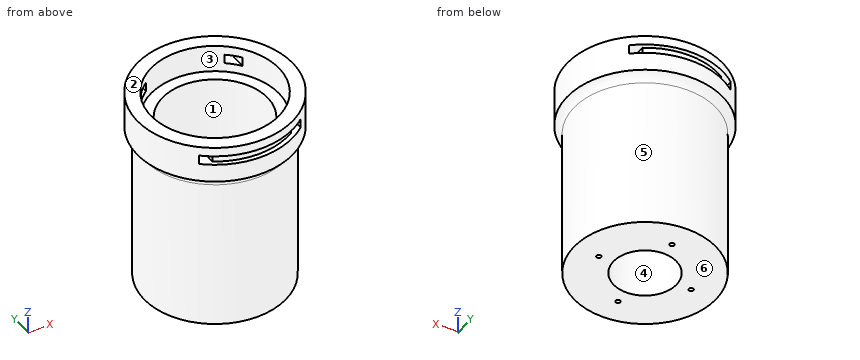
```python
from build123d import *

# Parameters (mm, degrees)
BOSS_EXTRUDE5_DEPTH      = 26
BOSS_EXTRUDE5_DEPTH_BACK = 17
SKETCH1_R                = 15.5
SKETCH3_R                = 5.625
CUT_EXTRUDE2_DEPTH       = 49.264894074
CUT_EXTRUDE3_DEPTH       = 28
CUT_EXTRUDE3_DEPTH_BACK  = 20
SKETCH4_R                = 11.5
CUT_EXTRUDE6_START       = 6
SKETCH7_R                = 11.5
SKETCH7_R_2              = 8.5
CUT_EXTRUDE6_DEPTH       = 18
BOSS_EXTRUDE8_DEPTH      = 6
BOSS_EXTRUDE8_DEPTH_BACK = 2
BOSS_EXTRUDE8_START      = 20
SKETCH12_R               = 17
CUT_EXTRUDE10_START      = 18
SKETCH13_R               = 11.5
CUT_EXTRUDE10_DEPTH      = 18.411862419
FILLET2_R                = 2
CUT_EXTRUDE11_START      = 26
SKETCH14_R               = 14
CUT_EXTRUDE11_DEPTH      = 6
CUT_EXTRUDE14_DEPTH      = 36.411862419
CUT_EXTRUDE14_DEPTH_BACK = 36.411862419
SKETCH15_R               = 0.5
SKETCH18_W               = 2.5
SKETCH18_H               = 2
CUT_EXTRUDE15_DEPTH      = 20
CUT_EXTRUDE16_DEPTH      = 2
SKETCH28_R               = 6.875
CUT_EXTRUDE17_DEPTH      = 16


with BuildPart() as part:
    # Sketch1 → Boss-Extrude5 (new, two sides: drawn at the far end of the back side and taken through both)
    with BuildSketch(Plane.XY.offset(-BOSS_EXTRUDE5_DEPTH_BACK)):
        Circle(SKETCH1_R)
    extrude(amount=BOSS_EXTRUDE5_DEPTH + BOSS_EXTRUDE5_DEPTH_BACK)

    # Sketch3 → Cut-Extrude2 (cut, through all)
    with BuildSketch(Plane.XY.offset(26)):
        Circle(SKETCH3_R)
    extrude(amount=-CUT_EXTRUDE2_DEPTH, mode=Mode.SUBTRACT)

    # Sketch4 → Cut-Extrude3 (cut, two sides: drawn at the far end of the back side and taken through both)
    with BuildSketch(Plane.XY.offset(26).offset(-CUT_EXTRUDE3_DEPTH_BACK)):
        Circle(SKETCH4_R)
    extrude(amount=CUT_EXTRUDE3_DEPTH + CUT_EXTRUDE3_DEPTH_BACK, mode=Mode.SUBTRACT)

    # Sketch7 → Cut-Extrude6 (cut)
    with BuildSketch(Plane.XY.offset(CUT_EXTRUDE6_START)):
        Circle(SKETCH7_R)
        Circle(SKETCH7_R_2, mode=Mode.SUBTRACT)
    extrude(amount=-CUT_EXTRUDE6_DEPTH, mode=Mode.SUBTRACT)

    # Sketch12 → Boss-Extrude8 (add, two sides: drawn at the far end of the back side and taken through both)
    with BuildSketch(Plane.XY.offset(BOSS_EXTRUDE8_START - BOSS_EXTRUDE8_DEPTH_BACK)):
        Circle(SKETCH12_R)
    extrude(amount=BOSS_EXTRUDE8_DEPTH + BOSS_EXTRUDE8_DEPTH_BACK)

    # Sketch13 → Cut-Extrude10 (cut, through all)
    with BuildSketch(Plane.XY.offset(CUT_EXTRUDE10_START)):
        Circle(SKETCH13_R)
    extrude(amount=CUT_EXTRUDE10_DEPTH, mode=Mode.SUBTRACT)

    # Fillet2
    # the kernel refuses this fillet: 2 mm, written as the material it adds along each edge
    with BuildSketch(Plane(origin=(0, 0, 18), x_dir=(1, 0, 0), z_dir=(0, 1, 0))) as fillet2_piece_1:
        with BuildLine():
            CenterArc((17.5, 1.936491673), FILLET2_R, 180, 75.522487814)
            Line((17, 0), (16.99, -0.038729833))
            ThreePointArc((16.99, -0.038729833), (16.25, -0.04), (15.5, -0.04))
            Line((15.5, -0.04), (15.46, 0))
            Line((15.46, 0), (15.46, 1.936491673))
            Line((15.46, 1.936491673), (15.5, 1.936491673))
        make_face()
    revolve(axis=Axis((0, 0, 18), (0, 0, -1)))

    # Sketch14 → Cut-Extrude11 (cut)
    with BuildSketch(Plane.XY.offset(CUT_EXTRUDE11_START)):
        Circle(SKETCH14_R)
    extrude(amount=-CUT_EXTRUDE11_DEPTH, mode=Mode.SUBTRACT)

    # Sketch15 → Cut-Extrude14 (cut, two sides: drawn at the far end of the back side and taken through both)
    with BuildSketch(Plane.XY.offset(-CUT_EXTRUDE14_DEPTH_BACK)):
        with Locations((0, 10)):
            Circle(SKETCH15_R)
        with Locations((0, -10)):
            Circle(SKETCH15_R)
        with Locations((10, 0)):
            Circle(SKETCH15_R)
        with Locations((-10, 0)):
            Circle(SKETCH15_R)
    extrude(amount=CUT_EXTRUDE14_DEPTH + CUT_EXTRUDE14_DEPTH_BACK, mode=Mode.SUBTRACT)

    # Sketch18 → Cut-Extrude15 (cut, symmetric)
    with BuildSketch(Plane(origin=(0, 0, 0), x_dir=(1, 0, 0), z_dir=(0, 1, 0))):
        with Locations((-9.75, -23)):
            Rectangle(SKETCH18_W, SKETCH18_H)
        with Locations((9.75, -23)):
            Rectangle(SKETCH18_W, SKETCH18_H)
    extrude(amount=CUT_EXTRUDE15_DEPTH, both=True, mode=Mode.SUBTRACT)

    # Sketch23 → Cut-Extrude16 (cut)
    with BuildSketch(Plane(origin=(0, 0, 24), x_dir=(-1, 0, 0), z_dir=(0, 0, -1))):
        with BuildLine():
            Line((9.719197711, 13.947659153), (9.147480199, 13.127208615))
            ThreePointArc((9.147480199, 13.127208615), (0, 16), (-9.147480199, 13.127208615))
            Line((-9.147480199, 13.127208615), (-9.719197711, 13.947659153))
            ThreePointArc((-9.719197711, 13.947659153), (0, 17), (9.719197711, 13.947659153))
        make_face()
        with BuildLine():
            Line((-9.147480199, -13.127208615), (-9.719197711, -13.947659153))
            ThreePointArc((-9.719197711, -13.947659153), (0, -17), (9.719197711, -13.947659153))
            Line((9.719197711, -13.947659153), (9.147480199, -13.127208615))
            ThreePointArc((9.147480199, -13.127208615), (0, -16), (-9.147480199, -13.127208615))
        make_face()
    extrude(amount=CUT_EXTRUDE16_DEPTH, mode=Mode.SUBTRACT)

    # Sketch28 → Cut-Extrude17 (cut)
    with BuildSketch(Plane(origin=(0, 0, -17), x_dir=(-1, 0, 0), z_dir=(0, 0, -1))):
        Circle(SKETCH28_R)
    extrude(amount=-CUT_EXTRUDE17_DEPTH, mode=Mode.SUBTRACT)


solid = part.part
```
The listing builds one solid part. Answer for the finished solid, in the listing's coordinates (mm). Face numbers are marked on the shaded views. A direction names the side the tool comes from. Coordinates: 2 decimals unless noted, no trailing zeros. Order: outer loops, then holes, each group sorted by start corner. A loop starts at its lowest first (then second) coordinate and runs counter-clockwise, first axis right, second up. Notation, with made-up numbers: M 32,14 L 88,14 A12 cw 88,22 Z; hole C -16.75,-10 d1. An arc over 180 degrees is marked long. Answer as a JSON object with one key per item and string values. Group by question number.
1. Determine the mould class of the marked faces 3, 4, 5 and 6 for opening direction Y: released by +Y, released by -Y, zero draft, split by the parting line, or undercut.
2. Straight lines are drawn through the part: line 1 (Y direction, x = 0, z = -11) (3 decimals); line 2 (X direction, y = -3, z = 0.5); line 3 (X direction, y = -11, z = 24.5). For each, find the intervals that lie inside material, in ascending order.
3. A tool of negligible diameter and unlimited length cuts with its end or side. For the marked faces 1 and 2, from which of +Z, -Z, +X, -X, +Y, -Y can it reach the whole face along a straight path? Write none if from no direction.
4. Flat-ended cylindrical pins translate along their axes: P1, Ø8.5, axis at x = 0, y = -1, coming from the +Z side; P2, Ø1, axis at x = 8, z = 8.5, coming from the +Y side; P3, Ø0.6, axis at y = 10, z = 23, coming from the -X side; P4, Ø1, axis at y = -12.5, z = 23.5, coming from the -X side. Find the tip coordinate at first contact, or state that the pin passes through.
5. Section A-A on z = -6.5 is taken. Write down the section's boundary in (x, y) (3 decimals), then the cut area to 3 significant figures.
6. Section B-B on z = 9 is taken. Write down the section's boundary in (x, y), then the cut area to 3 significant figures.
Values follow:
{
 "1": {"face 3": "undercut", "face 4": "undercut", "face 5": "split by the parting line", "face 6": "zero draft"},
 "2": {"line 1": "-15.5 to -11.5, -8.5 to -6.875, 6.875 to 8.5, 11.5 to 15.5", "line 2": "-15.21 to -11.1, -7.95 to -4.76, 4.76 to 7.95, 11.1 to 15.21", "line 3": "-12.96 to -8.66, 8.66 to 12.96"},
 "3": {"face 1": "+Z", "face 2": "+Z, +X, -X, +Y, -Y"},
 "4": {"P1": "through", "P2": "y = 13.56", "P3": "x = -13.96", "P4": "x = -12.04"},
 "5": {"outline": "C 0,0 d31; C 0,0 d17; hole C 0,0 d23; hole C 0,0 d13.75", "area": "418 mm2"},
 "6": {"outline": "C 0,0 d31; hole C 0,0 d23", "area": "339 mm2"}
}
